from build123d import *

# Parameters (mm, degrees)
BOSS_EXTRUDE2_DEPTH = 3


with BuildPart() as part:
    # Sketch4 → Boss-Extrude2 (new body)
    with BuildSketch(Plane(origin=(0, 0, 0), x_dir=(1, 0, 0), z_dir=(0, 1, 0))):
        Polygon((-26, -90), (-9.5, -90), (-9.5, -87), (15.5, -87), (15.5, -90), (32, -90), (32, -78), (29, -78), (29, -56), (32, -56), (32, -34), (29, -34), (29, -12), (32, -12), (32, 0), (15.5, 0), (15.5, -3), (-9.5, -3), (-9.5, 0), (-26, 0), (-26, -12), (-23, -12), (-23, -34), (-26, -34), (-26, -56), (-23, -56), (-23, -78), (-26, -78), align=None)
        with BuildLine():
            Line((-18.2, -61.3), (-5.8, -61.3))
            Line((-5.8, -61.3), (-5.8, -58.3))
            ThreePointArc((-5.8, -58.3), (1.3, -38.8), (-18.2, -31.7))
            Line((-18.2, -31.7), (-18.2, -61.3))
        make_face(mode=Mode.SUBTRACT)
        with BuildLine():
            ThreePointArc((4.693936025, -39.75), (0.374368671, -32.625631329), (-6.75, -28.306063975))
            ThreePointArc((-6.75, -28.306063975), (-12.308483212, -17.647580763), (-1.65, -12.089097551))
            ThreePointArc((-1.65, -12.089097551), (12.395183951, -20.604816049), (20.910902449, -34.65))
            ThreePointArc((20.910902449, -34.65), (15.352419237, -45.308483212), (4.693936025, -39.75))
        make_face(mode=Mode.SUBTRACT)
    extrude(amount=BOSS_EXTRUDE2_DEPTH)


solid = part.part
Source: CAD feature listing. Evaluate the final solid. Frame: model axes, mm. A direction names the side the tool comes from. Give positions to 0.01 mm unless a question says otherwise; leave off trailing zeros. Write each loop counter-clockwise with the first axis right and the second up, starting at its lowest first coordinate (ties: lowest second). Pieces come first, ordered by that corner, then holes. Notation, with made-up numbers: M 50,44 L 89,44 A14 ccw 89,65 Z; hole C -24.75,87 d9. An arc over 180 degrees is marked long. Answer as a JSON object with one key per item and string values.
Q1. Cut plane C-C, the plane y = 2.3. Count the separate pieces of the cut face and the enclosed holes in it, then the cut area to 3 significant figures.
Geometry check:
{"separate pieces": "1", "enclosed holes": "2", "area": "3,610 mm^2"}
Q2. Cut plane A-A, the plane z = 37.2. Return the cut outline in (x, y).
Geometry check:
{"outline": "M -26,0 L -18.2,0 L -18.2,3 L -26,3 Z; M 0.43,0 L 3.67,0 L 3.67,3 L 0.43,3 Z; M 21.3,0 L 32,0 L 32,3 L 21.3,3 Z"}
Q3. Access query for faces 1 (the face through (-9.5, 1, 89)), 2 (the face through (0.46, 1.48, 32.71)), 3 (the face through (-24, 1, 34)), 4 (the face through (30, 1, 12)). Directions: +Z, -Z, +X, -X, +Y, -Y. A direction counts if a zero-diameter tool reaches every point of the face in a straight line with its end or side. Return the directions, or none.
Geometry check:
{"face 1": "+Z, +Y, -Y", "face 2": "+Y, -Y", "face 3": "-X, +Y, -Y", "face 4": "+X, +Y, -Y"}
Q4. Cut plane D-D, the plane x = 8. Return the cut outline in (y, z), then the cut area to 3 significant figures.
Geometry check:
{"outline": "M 0,3 L 3,3 L 3,16.89 L 0,16.89 Z; M 0,44.21 L 3,44.21 L 3,87 L 0,87 Z", "area": "170 mm^2"}
Q5. Ray query, line 1 along X through (y, z) = (0.2, 41.5); line 2 along Z through (x, y) = (-5, 1.4); line 3 along X through (y, z) = (0.4, 39). Return the intervals inside material, ascending.
Geometry check:
{"line 1": "x = -26 to -18.2, 2.25 to 5.47, 20.13 to 32", "line 2": "z = 3 to 11.74, 28.96 to 32.1, 57.9 to 87", "line 3": "x = -26 to -18.2, 1.39 to 4.44, 21.11 to 32"}
Q6. Contact query for flat-ended pins moving along their axis: P1, Ø0.9, axis at y = 1, z = 67, coming from the +X side; P2, Ø0.9, axis at y = 1, z = 63.5, coming from the -X side. Output: stop coordinate, or through.
Geometry check:
{"P1": "stops at x = 29", "P2": "stops at x = -23"}
Q7. Mould query, pull axis X, two halves, no side actions, for faces 5 (the face through (9, 3, 54)), 6 (the face through (-23, 1, 67)), 7 (the face through (-5.8, 1, 60)). Classes: +X half, -X half, draft (parallel to the pull), parting line (faces both ways), or undercut.
Geometry check:
{"face 5": "draft", "face 6": "-X half", "face 7": "undercut"}
Q8. Cut plane B-B, the plane x = -4. Return the cut outline in (y, z), then the cut area to 3 significant figures.
Geometry check:
{"outline": "M 0,3 L 3,3 L 3,11.7 L 0,11.7 Z; M 0,29.44 L 3,29.44 L 3,32.7 L 0,32.7 Z; M 0,57.3 L 3,57.3 L 3,87 L 0,87 Z", "area": "125 mm^2"}
